Autodesk Inventor part; units mm, degrees
ref_plane "YZ Plane" through (0, 0, 0) normal (1, 0, 0) x (0, 1, 0)
ref_plane "XZ Plane" through (0, 0, 0) normal (0, 1, 0) x (-1, 0, 0)
ref_plane "XY Plane" through (0, 0, 0) normal (0, 0, 1) x (1, 0, 0)
sketch "Sketch1" plane through (0, 0, 0) normal (0, 1, 0) x (-1, 0, 0)
  line L0 (0, 0) -> (20.32, 0)
  line L1 (0, 101.6) -> (0, 0)
  line L2 (44.45, 76.2) -> (20.32, 76.2)
  line L3 (20.32, 76.2) -> (20.32, 101.6)
  line L4 (44.45, 76.2) -> (44.45, 25.4)
  line L5 (20.32, 101.6) -> (0, 101.6)
  line L6 (16.002, 88.9) -> (16.002, 76.2)
  line L7 (9.398, 76.2) -> (9.398, 88.9)
  arc A0 (16.002, 88.9) -> (9.398, 88.9) centre (12.7, 88.9) ccw
  arc A1 (9.398, 76.2) -> (16.002, 76.2) centre (12.7, 76.2) ccw
  line L8 (16.002, 25.4) -> (16.002, 12.7)
  line L9 (9.398, 12.7) -> (9.398, 25.4)
  arc A2 (16.002, 25.4) -> (9.398, 25.4) centre (12.7, 25.4) ccw
  arc A3 (9.398, 12.7) -> (16.002, 12.7) centre (12.7, 12.7) ccw
  line L10 (44.45, 25.4) -> (20.32, 25.4)
  line L11 (20.32, 25.4) -> (20.32, 0)
  dimension "d1" = 101.6
  dimension "d8" = 44.45
  dimension "d11" = 6.604
  dimension "d14" = 12.7
  dimension "d15" = 12.7
  dimension "d18" = 12.7
  dimension "d19" = 20.32
  dimension "d21" = 31.75
  dimension "d23" = 50.8
  dimension "d24" = 25.4
  dimension "d25" = 63.5
  dimension "d26" = 6.604
extrude "Extrusion1" add sketch "Sketch1" against normal blind 4.7625
fillet "Fillet1" radius 3.175 6 edges at (-20.32, -2.3813, 76.2) (-20.32, -2.3813, 101.6) (0, -2.3813, 101.6) (0, -2.3813, 0) (-20.32, -2.3813, 0) (-20.32, -2.3813, 25.4)
mirror "Mirror2" about plane through (-44.45, 0, 76.2) normal (-1, 0, 0)
equation "\"d26\" = d11"
properties part number "torchMount_back"
Design review of the part built by this model. Coordinates are the model's own, in mm. A direction names the side the tool comes from. Round coordinates to 2 decimals unless told otherwise and drop trailing zeros. Write each loop counter-clockwise with the first axis right and the second up, starting at its lowest first coordinate (ties: lowest second). Pieces come first, ordered by that corner, then holes. Notation, with made-up numbers: (44.25, 5) - (82.25, 5) arc R5 cw to (82.25, 11) - close; hole circle Ø5 at (-9, -18). An arc over 180 degrees is marked (long way). Use a Markdown table: item, result. Add a question column.
1. We need section A-A (x = -76.2). State the section outline as (y, z) points.
2. We need section B-B (z = 85). State the section outline as (x, y) points, then the cut area to 3 significant figures.
3. Mouldability with a two-part tool opening along Z and no side actions: class faces 1 (the face through (-12.6, -2.3, 9.4)), 2 (the face through (-20.32, -2, 13)), 3 (the face through (-87.95, -2.41, 100.69)) as +Z half, -Z half, draft (parallel to the pull), parting line (faces both ways), or undercut.
4. We need section C-C (z = 27). State the section outline as (x, y) points, then the cut area to 3 significant figures.
5. For faces 4 (the face through (-21.23, -2.41, 24.45)), 5 (the face through (-0.91, -2.41, 100.65)), 6 (the face through (-44, 0, 52)), 7 (the face through (-72.898, -2, 82)), 8 (the face through (-19, -2, 101)), list the 3-axis set-ups (+Z, -Z, +X, -X, +Y, -Y) from which the entire face can be reached by the end or side of a thin tool; tool diameter is ignored.
6. Wall thickness on probe 1 along X at (y, z) = (-4.25, 15); probe 2 along X at (y, z) = (-0.45, 77); probe 3 along X at (y, z) = (-3.75, 75.5): over which ranges is each line inside the solid? List them lowest first.
7. Clearance check with a flat-ended pin moving along its axis: pin 1 (2 mm diameter, centred on x = -60.5, y = -3, fed in from -Z). State where the tip first meets the part, or that it passes through.
8. We need section D-D (y = -2.45). Count the separate pieces of the cut face and the enclosed holes in it, then the cut area to 3 significant figures.
Output:
| question | item | result |
|---|---|---|
| 1 | outline | (-4.76, 0) - (0, 0) - (0, 9.4) - (-4.76, 9.4) - close; (-4.76, 28.7) - (0, 28.7) - (0, 72.9) - (-4.76, 72.9) - close; (-4.76, 92.2) - (0, 92.2) - (0, 101.6) - (-4.76, 101.6) - close |
| 2 | outline | (-88.9, -4.76) - (-79.5, -4.76) - (-79.5, 0) - (-88.9, 0) - close; (-72.9, -4.76) - (-68.58, -4.76) - (-68.58, 0) - (-72.9, 0) - close; (-20.32, -4.76) - (-16, -4.76) - (-16, 0) - (-20.32, 0) - close; (-9.4, -4.76) - (0, -4.76) - (0, 0) - (-9.4, 0) - close |
| 2 | area | 131 mm2 |
| 3 | face 1 | undercut |
| 3 | face 2 | draft |
| 3 | face 3 | +Z half |
| 4 | outline | (-88.9, -4.76) - (-79.09, -4.76) - (-79.09, 0) - (-88.9, 0) - close; (-73.31, -4.76) - (-15.59, -4.76) - (-15.59, 0) - (-73.31, 0) - close; (-9.81, -4.76) - (0, -4.76) - (0, 0) - (-9.81, 0) - close |
| 4 | area | 368 mm2 |
| 5 | face 4 | -Z, +Y, -Y |
| 5 | face 5 | +Z, +X, +Y, -Y |
| 5 | face 6 | +Z, -Z, +X, -X, +Y |
| 5 | face 7 | +Y, -Y |
| 5 | face 8 | +Z, +Y, -Y |
| 6 | probe 1 | x = -88.9 to -79.5, -72.9 to -68.58, -20.32 to -16, -9.4 to 0 |
| 6 | probe 2 | x = -88.9 to -79.5, -72.9 to -67.51, -21.39 to -16, -9.4 to 0 |
| 6 | probe 3 | x = -88.9 to -79.43, -72.97 to -15.93, -9.47 to 0 |
| 7 | pin 1 | stops at z = 25.4 |
| 8 | separate pieces | 1 |
| 8 | enclosed holes | 4 |
| 8 | area | 6,100 mm2 |
